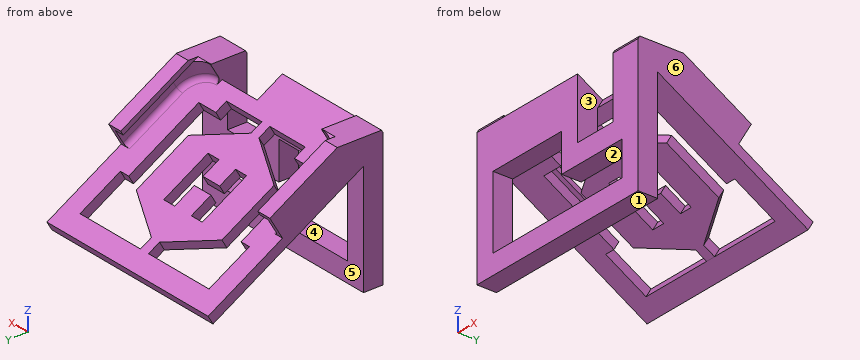
from build123d import *
from OCP.BRepFilletAPI import BRepFilletAPI_MakeChamfer

# Parameters (mm, degrees)
SKETCH1_W           = 80
SKETCH1_H           = 50
BOSS_EXTRUDE1_DEPTH = 8
BOSS_EXTRUDE2_DEPTH = 80
SKETCH3_W           = 2.1
SKETCH3_H           = 35
BOSS_EXTRUDE3_DEPTH = 8.3
FILLET1_R           = 10
FILLET2_R           = 2
BOSS_EXTRUDE4_DEPTH = 10
CHAMFER2_SIZE       = 17.320508076
CHAMFER2_SIZE_2     = 10
SKETCH5_W           = 12.5
SKETCH5_H           = 9.237604307
BOSS_EXTRUDE5_DEPTH = 8.3
SKETCH6_W           = 6
SKETCH6_H           = 47.309401077
BOSS_EXTRUDE6_DEPTH = 2
CHAMFER3_SIZE       = 9
CHAMFER3_SIZE2      = 15.588457268
SKETCH7_W           = 17.5
SKETCH7_H           = 11.773502692
CUT_EXTRUDE1_DEPTH  = 12
SKETCH8_W           = 17.5
SKETCH8_H           = 15
CUT_EXTRUDE2_DEPTH  = 12
CUT_EXTRUDE3_DEPTH  = 12
CUT_EXTRUDE4_DEPTH  = 4
BOSS_EXTRUDE7_DEPTH = 4
CUT_EXTRUDE5_REACH  = 87.126
SKETCH12_W          = 17.5
SKETCH12_H          = 2.535898385


with BuildPart() as part:
    # Sketch1 → Boss-Extrude1 (new body)
    with BuildSketch(Plane(origin=(0, 0, 0), x_dir=(1, 0, 0), z_dir=(0, 1, 0))):
        Rectangle(SKETCH1_W, SKETCH1_H)
    extrude(amount=BOSS_EXTRUDE1_DEPTH)

    # Sketch2 → Boss-Extrude2 (add)
    with BuildSketch(Plane(origin=(40, 0, 0), x_dir=(0, 0, -1), z_dir=(1, 0, 0))):
        Polygon((15, 69.282032303), (11.535898385, 71.282032303), (-25, 8), (-20.381197846, 8), align=None)
    extrude(amount=-BOSS_EXTRUDE2_DEPTH)

    # Sketch3 → Boss-Extrude3 (add)
    with BuildSketch(Plane(origin=(0, 12.825317547, 22.214101615), x_dir=(1, 0, 0), z_dir=(0, 0.5000000000000041, 0.8660254037844364))):
        with Locations((-38.95, 15)):
            Rectangle(SKETCH3_W, SKETCH3_H)
        Polygon((-27.5, -5.57179677), (-27.5, -2.5), (-37.9, -2.5), (-40, -2.5), (-40, -5.57179677), align=None)
        Polygon((40, -5.57179677), (40, -2.5), (37.9, -2.5), (27.5, -2.5), (27.5, -5.57179677), align=None)
        with Locations((38.95, 15)):
            Rectangle(SKETCH3_W, SKETCH3_H)
    extrude(amount=BOSS_EXTRUDE3_DEPTH)

    # Fillet1
    fillet1_edges = [part.edges().sort_by_distance(p)[0] for p in [
        (-37.9, 12.735254038, 27.058107041),
        (37.9, 12.735254038, 27.058107041),
    ]]
    fillet(fillet1_edges, radius=FILLET1_R)

    # Fillet2
    fillet2_edges = [part.edges().sort_by_distance(p)[0] for p in [
        (-27.7, 10.660254038, 23.464101615),
        (-37.9, 30.145825623, 12.214101615),
        (27.7, 10.660254038, 23.464101615),
        (37.9, 30.145825623, 12.214101615),
        (34.971067812, 13.196783719, 21.999635521),
        (-34.971067812, 13.196783719, 21.999635521),
    ]]
    fillet(fillet2_edges, radius=FILLET2_R)

    # Sketch4 → Boss-Extrude4 (add)
    with BuildSketch(Plane.XY.offset(25)):
        Polygon((40, 0), (40, 8), (27.5, 8), (-27.5, 8), (-40, 8), (-40, 0), align=None)
    extrude(amount=BOSS_EXTRUDE4_DEPTH)

    # Chamfer2
    # the kernel refuses this chamfer: 17.320508076, 10 mm, written as the material it takes off along each edge
    with BuildSketch(Plane(origin=(-84.809639706, 8, 35), x_dir=(0, -0.999813220622208, 0.019326765612700497), z_dir=(1, 0, 0))) as chamfer2_piece_1:
        Polygon((CHAMFER2_SIZE * 0.999813220604, CHAMFER2_SIZE * 0.0193267656124), (-CHAMFER2_SIZE_2 * 0.0193267656127, CHAMFER2_SIZE_2 * 0.999813220622), (0, 0), align=None)
    extrude(amount=169.619279412, mode=Mode.SUBTRACT)

    # Sketch5 → Boss-Extrude5 (add)
    with BuildSketch(Plane(origin=(0, 12.825317547, 22.214101615), x_dir=(1, 0, 0), z_dir=(0, 0.49999999999999656, 0.8660254037844407))):
        with Locations((-33.75, -10.190598924)):
            Rectangle(SKETCH5_W, SKETCH5_H)
        with Locations((33.75, -10.190598924)):
            Rectangle(SKETCH5_W, SKETCH5_H)
    extrude(amount=BOSS_EXTRUDE5_DEPTH)

    # Sketch6 → Boss-Extrude6 (add)
    with BuildSketch(Plane(origin=(0, 16.975317547, 29.402112467), x_dir=(1, 0, 0), z_dir=(0, 0.5000000000000041, 0.8660254037844364))):
        with Locations((-37, 8.845299461)):
            Rectangle(SKETCH6_W, SKETCH6_H)
        with Locations((37, 8.845299461)):
            Rectangle(SKETCH6_W, SKETCH6_H)
    extrude(amount=BOSS_EXTRUDE6_DEPTH)

    # Chamfer3: one chamfer whose edges measure the first distance from different faces: ONE call of the kernel's chamfer builder (chamfer() names one face for all edges)
    chamfer3_edges_1 = [part.edges().sort_by_distance(p)[0] for p in [
        (-37, 5.15, 38.538863812),
    ]]
    chamfer3_side_1 = [part.faces().sort_by_distance(p)[0] for p in [
        (-34.086933045, 2.341954644, 33.675186585),
    ]]
    chamfer3_edges_2 = [part.edges().sort_by_distance(p)[0] for p in [
        (37, 5.15, 38.538863812),
    ]]
    chamfer3_side_2 = [part.faces().sort_by_distance(p)[0] for p in [
        (34.086933045, 2.341954644, 33.675186585),
    ]]
    chamfer3 = BRepFilletAPI_MakeChamfer(part.part.solid().wrapped)
    for e in chamfer3_edges_1:
        chamfer3.Add(CHAMFER3_SIZE, CHAMFER3_SIZE2, e.wrapped, chamfer3_side_1[0].wrapped)  # the first distance lies on this face
    for e in chamfer3_edges_2:
        chamfer3.Add(CHAMFER3_SIZE, CHAMFER3_SIZE2, e.wrapped, chamfer3_side_2[0].wrapped)  # the first distance lies on this face
    add(Compound.cast(chamfer3.Shape()), mode=Mode.REPLACE)

    # Sketch7 → Cut-Extrude1 (cut)
    with BuildSketch(Plane(origin=(0, 12.825317547, 22.214101615), x_dir=(1, 0, 0), z_dir=(0, 0.49999999999999656, 0.8660254037844407))):
        with Locations((18.75, -8.922649731)):
            Rectangle(SKETCH7_W, SKETCH7_H)
    extrude(amount=-CUT_EXTRUDE1_DEPTH, mode=Mode.SUBTRACT)

    # Sketch8 → Cut-Extrude2 (cut)
    with BuildSketch(Plane(origin=(0, 8, 0), x_dir=(1, 0, 0), z_dir=(0, 1, 0))):
        with Locations((18.75, -12.42820323)):
            Rectangle(SKETCH8_W, SKETCH8_H)
    extrude(amount=-CUT_EXTRUDE2_DEPTH, mode=Mode.SUBTRACT)

    # Sketch9 → Cut-Extrude3 (cut)
    with BuildSketch(Plane(origin=(0, 8, 0), x_dir=(1, 0, 0), z_dir=(0, 1, 0))):
        Polygon((-32, -12.381197846), (2, -12.381197846), (2, 3.07179677), (32, 3.07179677), (32, 17), (-32, 17), align=None)
    extrude(amount=-CUT_EXTRUDE3_DEPTH, mode=Mode.SUBTRACT)

    # Sketch10 → Cut-Extrude4 (cut)
    with BuildSketch(Plane(origin=(0, 12.825317547, 22.214101615), x_dir=(1, 0, 0), z_dir=(0, 0.500000000000004, 0.8660254037844365))):
        Polygon((-19.5, 7.5), (-19.5, 2.42820323), (2, 2.42820323), (2, 4.964101615), (19.5, 4.964101615), (19.5, 7.5), (27.9, 7.5), (27.9, 40.5), (32, 40.5), (32, 59.5), (-32, 59.5), (-32, 40.5), (-27.9, 40.5), (-27.9, 7.5), align=None)
    extrude(amount=-CUT_EXTRUDE4_DEPTH, mode=Mode.SUBTRACT)

    # Sketch11 → Boss-Extrude7 (add)
    with BuildSketch(Plane(origin=(0, 12.825317547, 22.214101615), x_dir=(1, 0, 0), z_dir=(0, 0.500000000000004, 0.8660254037844365))):
        Polygon((-2, 32.140001961), (-2, 54.345299462), (-21.248711306, 43.232050808), (-21.248711306, 18.696152423), (-2, 7.582903769), (-2, 28.066803955), (-4.115553581, 28.066803955), (-4.115553581, 20.544526768), (-9.563712394, 20.544526768), (-9.563712394, 41.383676462), (-4.115553581, 41.383676462), (-4.115553581, 32.140001961), align=None)
        Polygon((21.248711306, 43.232050808), (2, 54.345299462), (2, 32.140001961), (4.115553581, 32.140001961), (4.115553581, 41.383676462), (9.563712394, 41.383676462), (9.563712394, 20.544526768), (4.115553581, 20.544526768), (4.115553581, 28.066803955), (2, 28.066803955), (2, 7.582903769), (21.248711306, 18.696152423), align=None)
        Polygon((2, 54.345299462), (0, 55.5), (-2, 54.345299462), (-2, 32.140001961), (0, 32.140001961), (2, 32.140001961), align=None)
        Polygon((-2, 54.345299462), (0, 55.5), (2, 54.345299462), (2, 59.5), (-2, 59.5), align=None)
        Polygon((0, 6.42820323), (-2, 7.582903769), (-2, 2.42820323), (2, 2.42820323), (2, 4.964101615), (2, 7.582903769), align=None)
        Polygon((0, 28.066803955), (-2, 28.066803955), (-2, 7.582903769), (0, 6.42820323), (2, 7.582903769), (2, 28.066803955), align=None)
    extrude(amount=-BOSS_EXTRUDE7_DEPTH)

    # Sketch12 → Cut-Extrude5 (cut, up to next)
    with BuildSketch(Plane(origin=(0, 12.825317547, 22.214101615), x_dir=(1, 0, 0), z_dir=(0, 0.500000000000004, 0.8660254037844365)), mode=Mode.PRIVATE) as cut_extrude5_sk1:
        with Locations((10.75, 3.696152423)):
            Rectangle(SKETCH12_W, SKETCH12_H)
    cut_extrude5_tool1 = extrude(cut_extrude5_sk1.sketch, amount=-CUT_EXTRUDE5_REACH, mode=Mode.PRIVATE) & part.part
    add(cut_extrude5_tool1.solids().sort_by_distance((10.75, 16.026279, 20.366025))[0], mode=Mode.SUBTRACT)


solid = part.part
Verification items for the finished model (mm, model axes). Face numbers are marked on the shaded views. A direction names the side the tool comes from. Give positions to 0.01 mm unless a question says otherwise; leave off trailing zeros. Write each loop counter-clockwise with the first axis right and the second up, starting at its lowest first coordinate (ties: lowest second). Pieces come first, ordered by that corner, then holes. Notation, with made-up numbers: (30.5, 84) -> (40.5, 84) arc R27 ccw to (40.5, 109) -> close; hole circle Ø4 at (21.25, -30.5). An arc over 180 degrees is marked (long way). Use CSV: the item, a comma, the result in double quotes.
(1) Material ranges on L1, parallel to X at y = 7, z = 7; L2, parallel to Y at x = 9.5, z = 16.5; L3, parallel to Y at x = 4, z = 20, recorded low to high.
Derived:
L1,"x = -40 to -32, 2 to 10, 27.5 to 40"
L2,"y = 0 to 8"
L3,"y = 0 to 8, 8.66 to 14.35"
(2) Go/stop test with flat-tipped pins: pin 1 (1.5 mm diameter, centred on x = 2.5, z = 14.5, fed in from +Y); pin 2 (6 mm diameter, centred on x = 21, z = 18, fed in from +Y); pin 3 (6 mm diameter, centred on x = -20.5, y = 43, fed in from -Z); pin 4 (3 mm diameter, centred on x = 20, z = -3.5, fed in from -Y). Record where each tip stops, or that it passes through.
Derived:
pin 1,"stops at y = 27.49"
pin 2,"stops at y = 19.32"
pin 3,"stops at z = -1.56"
pin 4,"stops at y = 0"
(3) Sectioned sample at D-D (y = 53). Record the cut outline in (x, z), plus the area to 3 significant figures.
Derived:
outline,"(-40, -5.6) -> (-32, -5.6) -> (-32, -0.98) -> (-40, -0.98) -> close; (-15.78, -0.98) -> (-11.78, -5.6) -> (11.78, -5.6) -> (15.78, -0.98) -> close; (32, -5.6) -> (40, -5.6) -> (40, -0.98) -> (32, -0.98) -> close"
area,"201 mm^2"
(4) Sectioned sample at A-A (z = -16). Record the cut outline in (x, y).
Derived:
outline,"(-40, 0) -> (-32, 0) -> (-32, 8) -> (-40, 8) -> close; (32, 0) -> (40, 0) -> (40, 8) -> (32, 8) -> close"
(5) Release check for a two-part mould opening along X. For the marked faces 4, 5 and 6 record: +X half, -X half, draft (parallel to the pull), parting line (faces both ways), or undercut.
Derived:
face 4,"undercut"
face 5,"draft"
face 6,"+X half"
(6) Sectioned sample at C-C (x = -15.5). Record the cut outline in (y, z), plus the area to 3 significant figures.
Derived:
outline,"(0, -25) -> (8, -25) -> (8, -17) -> (0, -17) -> close; (0, 12.38) -> (8, 12.38) -> (8, 20.38) -> (12.93, 17.54) -> (14.93, 21) -> (0, 29.62) -> close; (24.14, 11.06) -> (51.14, -4.53) -> (53.14, -1.06) -> (26.14, 14.53) -> close; (62.35, -11) -> (69.28, -15) -> (71.28, -11.54) -> (64.35, -7.54) -> close"
area,"368 mm^2"
(7) Set-up check for the marked faces 1, 2 and 3: record each of +Z, -Z, +X, -X, +Y, -Y from which the full face is reachable in a straight line by a thin tool's end or side.
Derived:
face 1,"-Z, +X, -X, +Y, -Y"
face 2,"-Y"
face 3,"+Z, -Y"
(8) Sectioned sample at B-B (x = 7). Record the cut outline in (y, z).
Derived:
outline,"(0, -25) -> (8, -25) -> (8, -17) -> (0, -17) -> close; (0, -3.07) -> (8, -3.07) -> (8, 20.38) -> (12.93, 17.54) -> (14.93, 21) -> (0, 29.62) -> close; (19.89, 13.52) -> (28.62, 8.48) -> (30.62, 11.94) -> (21.89, 16.98) -> close; (46.66, -1.94) -> (55.39, -6.98) -> (57.39, -3.52) -> (48.66, 1.52) -> close; (62.35, -11) -> (69.28, -15) -> (71.28, -11.54) -> (64.35, -7.54) -> close"
